Build history of the part. All positions in model axes, mm. A direction names the side the tool comes from. Give positions to 0.01 mm unless a question says otherwise; leave off trailing zeros. Order: outer loops, then holes, each group sorted by start corner. A loop starts at its lowest first (then second) coordinate and runs counter-clockwise, first axis right, second up. Notation, with made-up numbers: M 43.5,70 L 81.5,70 A20 cw 81.5,89 Z; hole C 9,-33 d3. An arc over 180 degrees is marked long. One line per item, written item: value. Start each with the question number.
from build123d import *

# Parameters (mm, degrees)
BOSS_EXTRUDE1_DEPTH = 5
BOSS_EXTRUDE2_DEPTH = 5
SKETCH3_R           = 1.625
CUT_EXTRUDE1_DEPTH  = 30


with BuildPart() as part:
    # Sketch1 → Boss-Extrude1 (new body)
    with BuildSketch(Plane(origin=(0, 0, 0), x_dir=(1, 0, 0), z_dir=(0, 1, 0))):
        with BuildLine():
            ThreePointArc((-4.815770235, 0), (-6.679809976, -4.500190024), (-11.18, -6.364229765))
            Line((-11.18, -6.364229765), (11.18, -6.364229765))
            ThreePointArc((11.18, -6.364229765), (4.815770235, 0), (11.18, 6.364229765))
            Line((11.18, 6.364229765), (-11.18, 6.364229765))
            ThreePointArc((-11.18, 6.364229765), (-6.679809976, 4.500190024), (-4.815770235, 0))
        make_face()
        with BuildLine():
            ThreePointArc((-11.18, 6.364229765), (-17.544229765, 0), (-11.18, -6.364229765))
            Line((-11.18, -6.364229765), (-11.18, -1.625))
            ThreePointArc((-11.18, -1.625), (-12.805, 0), (-11.18, 1.625))
            Line((-11.18, 1.625), (-11.18, 6.364229765))
        make_face()
        with BuildLine():
            Line((-11.18, -1.625), (-11.18, -6.364229765))
            ThreePointArc((-11.18, -6.364229765), (-6.679809976, -4.500190024), (-4.815770235, 0))
            ThreePointArc((-4.815770235, 0), (-6.679809976, 4.500190024), (-11.18, 6.364229765))
            Line((-11.18, 6.364229765), (-11.18, 1.625))
            ThreePointArc((-11.18, 1.625), (-10.030951481, 1.149048519), (-9.555, 0))
            ThreePointArc((-9.555, 0), (-10.030951481, -1.149048519), (-11.18, -1.625))
        make_face()
        with BuildLine():
            ThreePointArc((11.18, 6.364229765), (4.815770235, 0), (11.18, -6.364229765))
            Line((11.18, -6.364229765), (11.18, -1.625))
            ThreePointArc((11.18, -1.625), (9.555, 0), (11.18, 1.625))
            Line((11.18, 1.625), (11.18, 6.364229765))
        make_face()
        with BuildLine():
            Line((11.18, -1.625), (11.18, -6.364229765))
            ThreePointArc((11.18, -6.364229765), (15.680190024, -4.500190024), (17.544229765, 0))
            ThreePointArc((17.544229765, 0), (15.680190024, 4.500190024), (11.18, 6.364229765))
            Line((11.18, 6.364229765), (11.18, 1.625))
            ThreePointArc((11.18, 1.625), (12.329048519, 1.149048519), (12.805, 0))
            ThreePointArc((12.805, 0), (12.329048519, -1.149048519), (11.18, -1.625))
        make_face()
    extrude(amount=BOSS_EXTRUDE1_DEPTH)

    # Sketch2 → Boss-Extrude2 (add)
    with BuildSketch(Plane(origin=(0, 5, 0), x_dir=(1, 0, 0), z_dir=(0, 1, 0))):
        with BuildLine():
            Line((31.18, 6.364229765), (31.18, -6.364229765))
            Line((31.18, -6.364229765), (31.18, -57.387487167))
            add(Edge.make_bspline(
                [(31.18, -57.387487167), (37.440194103, -67.887046518), (46.22922531, -76.364229765)],
                knots=[0.492577267, 0.492577267, 0.492577267, 0.734976688, 0.734976688, 0.734976688], degree=2))
            Line((46.22922531, -76.364229765), (31.18, 6.364229765))
        make_face()
        with BuildLine():
            Line((31.18, -6.364229765), (16.18, -6.364229765))
            add(Edge.make_bspline(
                [(16.18, -6.364229765), (18.458726646, -36.051445121), (31.18, -57.387487167)],
                knots=[0, 0, 0, 0.492577267, 0.492577267, 0.492577267], degree=2))
            Line((31.18, -57.387487167), (31.18, -6.364229765))
        make_face()
        with BuildLine():
            Line((11.18, -6.364229765), (31.18, -6.364229765))
            Line((31.18, -6.364229765), (31.18, 6.364229765))
            Line((31.18, 6.364229765), (11.18, 6.364229765))
            ThreePointArc((11.18, 6.364229765), (17.544229765, 0), (11.18, -6.364229765))
        make_face()
    extrude(amount=-BOSS_EXTRUDE2_DEPTH)

    # Sketch3 → Cut-Extrude1 (cut)
    with BuildSketch(Plane(origin=(0, 5, 0), x_dir=(1, 0, 0), z_dir=(0, 1, 0))):
        with Locations((27.4505743, -12.246247431)):
            Circle(SKETCH3_R)
        with Locations((31.924922619, -36.842592833)):
            Circle(SKETCH3_R)
    extrude(amount=-CUT_EXTRUDE1_DEPTH, mode=Mode.SUBTRACT)


solid = part.part
1) Slice it at B-B (y = 3.95). State how many separate pieces and enclosed holes the cut face has, plus the area to 3 significant figures.
2) Drill centre lines: line 1 (Z direction, x = 2, y = 1.9); line 2 (Z direction, x = -11.5, y = 2.2); line 3 (Z direction, x = 31, y = 4.3). Where is each one in solid material? Low to high.
3) Tool access for faces 4 (the flat face through (10, 3, -6.364)), 5 (the flat face through (2, 3, 6.364)): list every direction of +Z, -Z, +X, -X, +Y, -Y with a clear straight run to the whole face (end or side of a thin tool).
4) Drop flat-ended pins along their axis: P1, Ø1, axis at y = 4, z = 23.5, coming from the +X side; P2, Ø2.5, axis at x = 0.5, y = 2.5, coming from the +Z side; P3, Ø1.5, axis at y = 2.5, z = 49.5, coming from the -X side. Give the stop position or say it passes through.
5) Pull direction X, two halves, no side cores. Call faces 1 (the flat face through (21, 0, 19)), 2 (the cylindrical face through (-17.543, 2.465, -0.14)), 3 (the cylindrical face through (26.3, 2.5, 11.1)): pulls with the +X half, pulls with the -X half, needs draft (parallel to the pull), parting line crosses it, or undercut.
6) Slice it at A-A (x = 4.5). List the corners of the cut face in (y, z), plus the area to 3 significant figures.
Results list:
1. separate pieces: 1
1. enclosed holes: 4
1. area: 1,550 mm²
2. line 1: z = -6.36 to 6.36
2. line 2: z = -6.36 to -1.59, 1.59 to 6.36
2. line 3: z = -6.36 to 35.51, 38.18 to 57.08
3. face 4: -Z, +X, -X, +Y, -Y
3. face 5: +Z, -X, +Y, -Y
4. P1: stops at x = 36.7
4. P2: stops at z = 6.36
4. P3: stops at x = 26.62
5. face 1: needs draft
5. face 2: pulls with the -X half
5. face 3: undercut
6. outline: M 0,-6.36 L 5,-6.36 L 5,6.36 L 0,6.36 Z
6. area: 63.6 mm²
